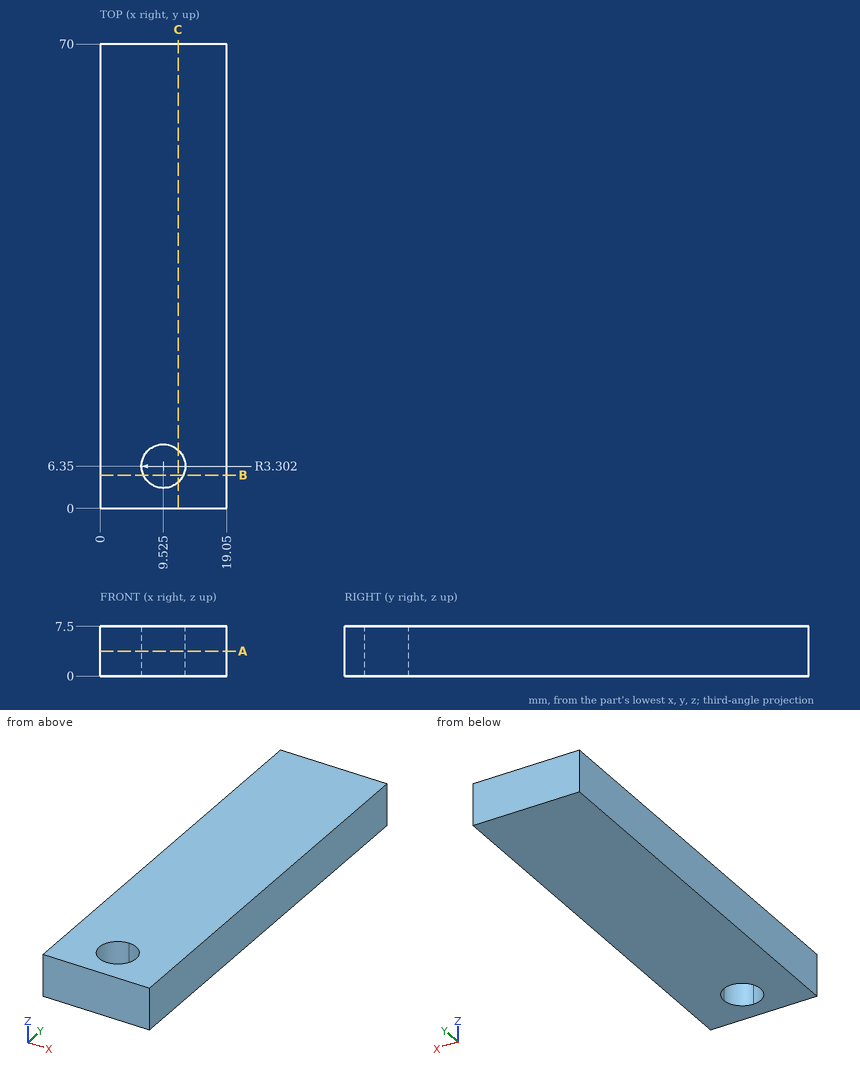
Study the drawing (mm; zero at the part's minimum x, y, z) and answer. Give positions to 0.01 mm unless a question says otherwise; leave off trailing zeros. Loops run counter-clockwise (first coordinate to the right, second up) from the corner with the lowest first, then second, coordinate; pieces in that order, holes last. Notation, with made-up numbers: (-20.5, 82.5) - (11.5, 82.5) arc R27 ccw to (11.5, 112.5) - close; hole circle Ø9 at (60.25, 48). An arc over 180 degrees is marked (long way). Answer as CSV lines item,"result". Start each with the question number.
1) Straight lines are drawn through the part: L1, parallel to X at y = 4.5, z = 2.25; L2, parallel to Y at x = 12.5, z = 4.5; L3, parallel to Y at x = 11, z = 7. For each, find the intervals that lie inside material, in ascending order. Write a range as from..to.
2) Find section A-A (z = 3.75). Write down the section's boundary in (x, y) (3 decimals).
3) Find section C-C (x = 11.75). Write down the section's boundary in (y, z).
4) This flat-tipped pin is pushed along its axis until it touches: pin 1 Ø4 at (x, y) = (4.5, 59) entering from -Z. Where does it stop, or does it pass through?
5) Find section B-B (y = 5). Write down the section's boundary in (x, z), then the cut area to 3 significant figures.
Findings below:
1,L1,"0..6.79, 12.26..19.05"
1,L2,"0..4.92, 7.78..70"
1,L3,"0..3.4, 9.3..70"
2,outline,"(0, 0) - (19.05, 0) - (19.05, 70) - (0, 70) - close; hole (9.525, 3.048) arc R3.302 ccw to (12.827, 6.35) arc R3.302 ccw (long way) to start"
3,outline,"(0, 0) - (3.91, 0) - (3.91, 7.5) - (0, 7.5) - close; (8.79, 0) - (70, 0) - (70, 7.5) - (8.79, 7.5) - close"
4,pin 1,"z = 0"
5,outline,"(0, 0) - (6.51, 0) - (6.51, 7.5) - (0, 7.5) - close; (12.54, 0) - (19.05, 0) - (19.05, 7.5) - (12.54, 7.5) - close"
5,area,"97.7 mm^2"
